Autodesk Inventor part; units mm, degrees
ref_plane "Work Plane1" through (27.8701, 0, -3.6069) normal (0, 0, -1) x (-1, 0, 0)
ref_plane "YZ Plane" through (0, 0, 0) normal (1, 0, 0) x (0, 1, 0)
ref_plane "XZ Plane" through (0, 0, 0) normal (0, 1, 0) x (-1, 0, 0)
sketch "Sketch1" plane through (0, 0, 0) normal (0, 1, 0) x (-1, 0, 0)
  line L0 (34.1299, -113.6069) -> (-27.8701, -113.6069)
  line L1 (-27.8701, -113.6069) -> (-27.8701, 106.3931)
  line L2 (-27.8701, 106.3931) -> (34.1299, 106.3931)
  line L3 (34.1299, 106.3931) -> (34.1299, -113.6069)
  line L4 (34.1299, -113.6069) -> (-27.8701, 106.3931) construction
  line L5 (-27.8701, -113.6069) -> (34.1299, 106.3931) construction
  point P0 (0, 0)
  point P1 (3.1299, -3.6069)
  dimension "d0" = 62
  dimension "d1" = 220
extrude "Extrusion1" add sketch "Sketch1" along normal blind 31.8
sketch "Sketch2" plane through (-34.1299, 0, 106.3931) normal (0, 0, 1) x (1, 0, 0)
  line L0 (62, 0) -> (0, 0)
  line L1 (62, 0) -> (62, 31.8)
  line L2 (0, 0) -> (0, 31.8)
  line L3 (2.8, 38.8076) -> (59.2, 38.8076)
  line L4 (59.2, 38.8076) -> (59.2, 2)
  line L5 (59.2, 2) -> (2.8, 2)
  line L6 (2.8, 2) -> (2.8, 38.8076)
  point P0 (34.1299, 0)
  dimension "d4" = 2.8
  dimension "d5" = 2.8
  dimension "d6" = 2
extrude "Extrusion2" cut sketch "Sketch2" against normal blind 12
ref_plane "Work Plane1" through (27.8701, 0, -3.6069) normal (0, 0, -1) x (-1, 0, 0)
mirror "Mirror1" about plane through (27.8701, 0, -3.6069) normal (0, 0, -1) of "Extrusion2"
sketch "Sketch3" plane through (0, 0, 0) normal (0, -1, 0) x (1, 0, 0)
  line L0 (-34.1299, -113.6069) -> (27.8701, -113.6069)
  line L1 (27.8701, -113.6069) -> (27.8701, 106.3931)
  line L2 (27.8701, 106.3931) -> (-34.1299, 106.3931)
  line L3 (-34.1299, 106.3931) -> (-34.1299, -113.6069)
  line L4 (-26.6299, 106.3931) -> (-26.6299, 102.8931)
  circle A0 centre (-26.6299, 102.8931) radius 1.5
  line L5 (-28.1299, 102.8931) -> (-28.1299, 106.3931)
  line L6 (-25.1299, 102.8931) -> (-25.1299, 106.3931)
  line L7 (20.3701, 106.3931) -> (20.3701, 102.8931)
  circle A1 centre (20.3701, 102.8931) radius 1.5
  line L8 (21.8701, 102.8931) -> (21.8701, 106.3931)
  line L9 (18.8701, 102.8931) -> (18.8701, 106.3931)
  line L10 (-26.6299, -113.6069) -> (-26.6299, -110.1069)
  circle A2 centre (-26.6299, -110.1069) radius 1.5
  line L11 (-25.1299, -110.1069) -> (-25.1299, -113.6069)
  line L12 (-28.1299, -110.1069) -> (-28.1299, -113.6069)
  line L13 (20.3701, -113.6069) -> (20.3701, -110.1069)
  circle A3 centre (20.3701, -110.1069) radius 1.5
  line L14 (18.8701, -110.1069) -> (18.8701, -113.6069)
  line L15 (21.8701, -110.1069) -> (21.8701, -113.6069)
  point P0 (0, 0)
  dimension "d9" = 3
  dimension "d10" = 3.5
  dimension "d11" = 6
  dimension "d12" = 3.5
  dimension "d14" = 3
  dimension "d15" = 3.5
  dimension "d16" = 3
  dimension "d18" = 3.5
  dimension "d19" = 3
  dimension "d23" = 6
  dimension "d24" = 6
  dimension "d25" = 6
extrude "Extrusion3" cut sketch "Sketch3" against normal blind 12 contours L12 A2 L10 L0 | L10 A2 L11 L0 | A2 | L2 L4 A0 L5 | L2 L6 A0 L4 | A0 | L14 A3 L13 L0 | L13 A3 L15 L0 | A3 | L2 L7 A1 L9 | L2 L8 A1 L7 | A1
properties part number "5v_psu"
Can you work these out from the model? Positions are in its coordinate system, mm. A direction names the side the tool comes from. Give positions to 0.01 mm unless a question says otherwise; leave off trailing zeros. Loops run counter-clockwise (first coordinate to the right, second up) from the corner with the lowest first, then second, coordinate; pieces in that order, holes last. Notation, with made-up numbers: (32, 83.25) -> (44, 83.25) arc R19 ccw to (44, 111.25) -> close; hole circle Ø2 at (88, 23). An arc over 180 degrees is marked (long way). Return JSON: item names as keys, results as strings.
Q1. I need wall thicknesses on probe 1 along Z at (x, y) = (-22, 11.5). Which ranges of the line are inside material? Lowest first, please.
Checks:
{"probe 1": "z = -101.61 to 94.39"}
Q2. For pin 1 Ø8 at (x, y) = (12.5, 21) entering from +Z; pin 2 Ø9.5 at (x, z) = (3, -106.5) entering from +Y; pin 3 Ø4 at (x, y) = (5.5, 10) entering from -Z, each with a flat end and sliding along its axis, tell me the tip position at first contact or that it passes through.
Checks:
{"pin 1": "stops at z = 94.39", "pin 2": "stops at y = 2", "pin 3": "stops at z = -101.61"}
Q3. On a 3-axis mill with a long thin cutter (end or side, diameter ignored), from which of +Z, -Z, +X, -X, +Y, -Y can I reach the whole of each face in a straight line? I mean faces 1 (the face through (-31.33, 17, 100)), 2 (the face through (-3, 31.8, -27)), 3 (the face through (-4, 2, -108)). Say none if no direction works.
Checks:
{"face 1": "+Z, +Y", "face 2": "+Z, -Z, +X, -X, +Y", "face 3": "-Z, +Y"}
Q4. I want a section at B-B, the plane x = 3. List the corners of the cut face in (y, z) for me.
Checks:
{"outline": "(0, -113.61) -> (2, -113.61) -> (2, -101.61) -> (31.8, -101.61) -> (31.8, 94.39) -> (2, 94.39) -> (2, 106.39) -> (0, 106.39) -> close"}
Q5. I want a section at A-A, the plane y = 22. List the corners of the cut face in (x, z) for me.
Checks:
{"outline": "(-34.13, -113.61) -> (-31.33, -113.61) -> (-31.33, -101.61) -> (25.07, -101.61) -> (25.07, -113.61) -> (27.87, -113.61) -> (27.87, 106.39) -> (25.07, 106.39) -> (25.07, 94.39) -> (-31.33, 94.39) -> (-31.33, 106.39) -> (-34.13, 106.39) -> close"}
